from build123d import *

# Parameters (mm, degrees)
SKETCH2_R           = 8.21
SKETCH2_R_2         = 6.235
BOSS_EXTRUDE1_DEPTH = 6.99
CUT_EXTRUDE3_START  = -2
SKETCH3_R           = 8.21
SKETCH3_R_2         = 6.235
CUT_EXTRUDE3_DEPTH  = 2
BOSS_EXTRUDE2_START = 2
SKETCH4_R           = 8.21
SKETCH4_R_2         = 6.235
BOSS_EXTRUDE2_DEPTH = 2
SKETCH7_R           = 8.21
SKETCH7_R_2         = 6.235
CUT_EXTRUDE4_DEPTH  = 2


with BuildPart() as part:
    # Sketch2 → Boss-Extrude1 (new body)
    with BuildSketch(Plane.XY):
        Circle(SKETCH2_R)
        Circle(SKETCH2_R_2, mode=Mode.SUBTRACT)
    extrude(amount=BOSS_EXTRUDE1_DEPTH)

    # Sketch3 → Cut-Extrude3 (cut)
    with BuildSketch(Plane.XY.offset(6.99).offset(CUT_EXTRUDE3_START)):
        Circle(SKETCH3_R)
        Circle(SKETCH3_R_2, mode=Mode.SUBTRACT)
    extrude(amount=CUT_EXTRUDE3_DEPTH, mode=Mode.SUBTRACT)

    # Sketch4 → Boss-Extrude2 (add)
    with BuildSketch(Plane(origin=(0, 0, 0), x_dir=(-1, 0, 0), z_dir=(0, 0, -1)).offset(BOSS_EXTRUDE2_START)):
        Circle(SKETCH4_R)
        Circle(SKETCH4_R_2, mode=Mode.SUBTRACT)
    extrude(amount=-BOSS_EXTRUDE2_DEPTH)

    # Sketch7 → Cut-Extrude4 (cut)
    with BuildSketch(Plane(origin=(0, 0, -2), x_dir=(-1, 0, 0), z_dir=(0, 0, -1))):
        Circle(SKETCH7_R)
        Circle(SKETCH7_R_2, mode=Mode.SUBTRACT)
    extrude(amount=-CUT_EXTRUDE4_DEPTH, mode=Mode.SUBTRACT)


solid = part.part
For this review, take the finished solid that the model builds, in its own axes (mm). Coordinates: 2 decimals unless noted, no trailing zeros. Loops run counter-clockwise (first coordinate to the right, second up) from the corner with the lowest first, then second, coordinate; pieces in that order, holes last. Notation, with made-up numbers: (-40, 29.5) - (-8, 29.5) arc R13 ccw to (-8, 36.5) - close; hole circle Ø6 at (16.5, 79). An arc over 180 degrees is marked (long way). Use a Markdown table: item, result. Add a question column.
Item 1: We need section A-A (y = 0). Give the boundary of the cut face in (x, z) (3 decimals), and give its area (3 significant figures).
Item 2: For line 1 (Y direction, x = 0, z = 3.5) (3 decimals); line 2 (Y direction, x = 3.75, z = 1.7); line 3 (X direction, y = 2.25, z = 1.35), list the stretches that pass through material, from the lowest coordinate up.
Item 3: We need section D-D (x = 7.25). Give the boundary of the cut face in (y, z).
Item 4: We need section C-C (z = 3.75). Give the boundary of the cut face in (x, y) (3 decimals), and give its area (3 significant figures).
Item 5: Insertion check: pin 1 Ø6 at (x, y) = (-5.5, -6.5) entering from +Z. The pin has a flat end and moves straight along its axis. Give the tip position at first contact, or say it passes through.
Item 6: Mouldability with a two-part tool opening along X and no side actions: class faces 1 (the face through (-1.78, -8.015, 2.46)), 2 (the face through (-1.352, -6.087, 2.46)), 3 (the face through (6, -3, 0)) as pulls with the +X half, pulls with the -X half, needs draft (parallel to the pull), parting line crosses it, or undercut.
Results list:
| question | item | result |
|---|---|---|
| 1 | outline | (-8.21, 0) - (-6.235, 0) - (-6.235, 4.99) - (-8.21, 4.99) - close; (6.235, 0) - (8.21, 0) - (8.21, 4.99) - (6.235, 4.99) - close |
| 1 | area | 19.7 mm^2 |
| 2 | line 1 | y = -8.21 to -6.235, 6.235 to 8.21 |
| 2 | line 2 | y = -7.3 to -4.98, 4.98 to 7.3 |
| 2 | line 3 | x = -7.9 to -5.81, 5.81 to 7.9 |
| 3 | outline | (-3.85, 0) - (3.85, 0) - (3.85, 4.99) - (-3.85, 4.99) - close |
| 4 | outline | circle Ø16.42 at (0, 0); hole circle Ø12.47 at (0, 0) |
| 4 | area | 89.6 mm^2 |
| 5 | pin 1 | stops at z = 4.99 |
| 6 | face 1 | parting line crosses it |
| 6 | face 2 | undercut |
| 6 | face 3 | needs draft |
